Design review of the part built by this model. Coordinates are the model's own, in mm. Give positions to 0.01 mm unless a question says otherwise; leave off trailing zeros. Order: outer loops, then holes, each group sorted by start corner. A loop starts at its lowest first (then second) coordinate and runs counter-clockwise, first axis right, second up. Notation, with made-up numbers: M -15.75,70 L -10.75,70 A23 ccw -10.75,84 Z; hole C -31.5,58.5 d9. An arc over 180 degrees is marked long. Put each result on its own line as item: value. Start each with the question number.
from build123d import *

# Parameters (mm, degrees)
F0_W        = 10
F0_H        = 20
F1_DEPTH    = 3
F2_R        = 2
F2_R_2      = 1.5
F3_DEPTH    = 3.001
F4_T1_DEPTH = 28
F4_T3_DEPTH = 42.9128784748


# Not quite as in the source:
# - a fillet or chamfer that OpenCascade refuses, or shapes differently, is made with other operations: its cross-section is extruded or revolved along the edge and cut away or added


with BuildPart() as f1:
    # F0 (on Front) → F1 (new body)
    with BuildSketch(Plane.XZ):
        with Locations((-0.1535092495, 0.14802441)):
            Rectangle(F0_W, F0_H)
    extrude(amount=F1_DEPTH)

    # F2 (on face) → F3 (cut, through all)
    with BuildSketch(Plane.XZ.offset(3)):
        with Locations((0, 7.14802441)):
            Circle(F2_R)
        with Locations((0, -6.85197559)):
            Circle(F2_R_2)
    extrude(amount=-F3_DEPTH, mode=Mode.SUBTRACT)

    # F4: fillet of radius 5 on 4 edges, made by hand

    # F4_s2 → F4_t1 (cut)
    with BuildSketch(Plane.XZ.offset(-12.5)):
        with BuildLine():
            ThreePointArc((4.8464907505, 5.14802441), (3.3820246565, 8.6835583159), (-0.1535092495, 10.14802441))
            Line((-0.1535092495, 10.14802441), (4.8464907505, 10.14802441))
            Line((4.8464907505, 10.14802441), (4.8464907505, 5.14802441))
        make_face()
        with BuildLine():
            ThreePointArc((-5.1535092495, 5.14802441), (-3.6890431554, 8.6835583159), (-0.1535092495, 10.14802441))
            Line((-0.1535092495, 10.14802441), (-5.1535092495, 10.14802441))
            Line((-5.1535092495, 10.14802441), (-5.1535092495, 5.14802441))
        make_face()
    extrude(amount=F4_T1_DEPTH, mode=Mode.SUBTRACT)

    # F4_s4 → F4_t3 (cut)
    with BuildSketch(Plane.XY.offset(-21.3084148274)):
        with BuildLine():
            ThreePointArc((-5.1535092495, 0), (-3.309546342, -2.1833001327), (-0.5709335545, -3))
            Line((-0.5709335545, -3), (-5.1535092495, -3))
            Line((-5.1535092495, -3), (-5.1535092495, 0))
        make_face()
        with BuildLine():
            ThreePointArc((4.8464907505, 0), (3.0025278431, -2.1833001327), (0.2639150556, -3))
            Line((0.2639150556, -3), (4.8464907505, -3))
            Line((4.8464907505, -3), (4.8464907505, 0))
        make_face()
    extrude(amount=F4_T3_DEPTH, mode=Mode.SUBTRACT)


solid = f1.part
1. The part is to be moulded in two halves that separate along X. For faces 1 (the cylindrical face through (-2, -1.5, 7.2)), 2 (the cylindrical face through (3.04, -2.16, 0)), 3 (the flat face through (0, 0, 0)), say which applies: +X half, -X half, draft (parallel to the pull), parting line (faces both ways), or undercut.
2. Consider section B-B on x = -2.5. Give the boundary of the cut face in (y, z).
3. To check wall thickness, follow probe 1 along Z at (x, y) = (0, -0.9); probe 2 along Z at (x, y) = (-0.75, -1.4); probe 3 along X at (y, z) = (-1.95, -5.5). State the ranges of each line that lie inside material, in increasing order.
4. Consider section A-A on y = -2.1. Give the boundary of the cut face in (x, z).
5. Consider section C-C on z = 4.25. Give the boundary of the cut face in (x, y).
6. Insertion check: pin 1 (1 mm diameter, centred on y = -2, z = 6, fed in from +X). The pin has a flat end and moves straight along its axis. Give the tip position at first contact, or say it passes through.
Returned:
1. face 1: undercut
1. face 2: +X half
1. face 3: draft
2. outline: M -2.61,-9.85 L 0,-9.85 L 0,9.56 L -2.61,9.56 Z
3. probe 1: z = -9.85 to -8.35, -5.35 to 5.15, 9.15 to 10.15
3. probe 2: z = -9.85 to -8.15, -5.55 to 5.29, 9 to 10.11
3. probe 3: x = -3.64 to -0.65, 0.65 to 3.33
4. outline: M -3.43,-9.85 L 3.13,-9.85 L 3.13,8.92 A5 ccw -3.43,8.92 Z; hole C 0,7.15 d4; hole C 0,-6.85 d3
5. outline: M -5.15,0 A5 ccw -0.57,-3 L 0.26,-3 A5 ccw 4.85,0 Z
6. pin 1: stops at x = 3.83
